from build123d import *

# Parameters (mm, degrees)
SKETCH1_W                  = 50.8
SKETCH1_H                  = 63.5
BOSS_EXTRUDE1_DEPTH        = 12.7
F_22_0_22_DIAMETER_HOLE1_D = 22
F_4_40_TAPPED_HOLE1_D      = 2.2606
CUT_EXTRUDE1_DEPTH         = 43.597094971
CUT_EXTRUDE2_DEPTH         = 6.35


with BuildPart() as part:
    # Sketch1 → Boss-Extrude1 (new body)
    with BuildSketch(Plane(origin=(0, 0, 0), x_dir=(0, 0, -1), z_dir=(1, 0, 0))):
        Rectangle(SKETCH1_W, SKETCH1_H)
    extrude(amount=BOSS_EXTRUDE1_DEPTH)

    # Ø22.0 (22) Diameter Hole1 (through all)
    with Locations(Plane(origin=(12.7, 0, 0), x_dir=(0, 0, -1), z_dir=(1, 0, 0))):
        with Locations((0, -12.7)):
            Hole(F_22_0_22_DIAMETER_HOLE1_D / 2)

    # Sketch4 → 1/16 NPT Tapped Hole1 (revolve, cut)
    with BuildSketch(Plane.ZX.offset(12.7)):
        Polygon((0, 0), (0, 13.530685027), (3.0734, 11.684), (3.0734, 6.858), (3.762574096, 6.858), (3.9679118, 0), align=None)
    revolve(axis=Axis((-6.35, 12.7, 0), (1, 0, 0)), mode=Mode.SUBTRACT)

    # #4-40 Tapped Hole1 (through all)
    with Locations(Plane(origin=(12.7, 0, 0), x_dir=(0, 0, -1), z_dir=(1, 0, 0))):
        with Locations((-12.5, 12.7), (12.5, 12.7)):
            Hole(F_4_40_TAPPED_HOLE1_D / 2)

    # Sketch9 → Cut-Extrude1 (cut, through all)
    with BuildSketch(Plane(origin=(12.7, 0, 0), x_dir=(0, 0, -1), z_dir=(1, 0, 0))):
        with BuildLine():
            Line((-3.65, 2.54), (3.65, 2.54))
            ThreePointArc((3.65, 2.54), (8.140128061, 4.399871939), (10, 8.89))
            Line((10, 8.89), (10, 16.51))
            ThreePointArc((10, 16.51), (8.140128061, 21.000128061), (3.65, 22.86))
            Line((3.65, 22.86), (-3.65, 22.86))
            ThreePointArc((-3.65, 22.86), (-8.140128061, 21.000128061), (-10, 16.51))
            Line((-10, 16.51), (-10, 8.89))
            ThreePointArc((-10, 8.89), (-8.140128061, 4.399871939), (-3.65, 2.54))
        make_face()
    extrude(amount=-CUT_EXTRUDE1_DEPTH, mode=Mode.SUBTRACT)

    # Sketch10 → Cut-Extrude2 (cut)
    with BuildSketch(Plane(origin=(0, 0, 0), x_dir=(0, 0, -1), z_dir=(1, 0, 0))):
        with BuildLine():
            Line((-12.5, 2.54), (12.5, 2.54))
            ThreePointArc((12.5, 2.54), (16.990128061, 4.399871939), (18.85, 8.89))
            Line((18.85, 8.89), (18.85, 16.51))
            ThreePointArc((18.85, 16.51), (16.990128061, 21.000128061), (12.5, 22.86))
            Line((12.5, 22.86), (-12.5, 22.86))
            ThreePointArc((-12.5, 22.86), (-16.990128061, 21.000128061), (-18.85, 16.51))
            Line((-18.85, 16.51), (-18.85, 8.89))
            ThreePointArc((-18.85, 8.89), (-16.990128061, 4.399871939), (-12.5, 2.54))
        make_face()
    extrude(amount=CUT_EXTRUDE2_DEPTH, mode=Mode.SUBTRACT)


solid = part.part
Part model, mm, in its own coordinate system. A direction names the side the tool comes from. Round coordinates to 2 decimals unless told otherwise and drop trailing zeros. Write each loop counter-clockwise with the first axis right and the second up, starting at its lowest first coordinate (ties: lowest second). Pieces come first, ordered by that corner, then holes. Notation, with made-up numbers: M -18.5,-26.75 L 24.5,-26.75 A30 ccw 24.5,3.25 Z; hole C 80.25,10.25 d11. An arc over 180 degrees is marked long. Return JSON: item names as keys, results as strings. Group by question number.
(1) Saw through at C-C on x = 11.75. Write the cut outline in (y, z).
(2) Saw through at B-B on y = -12.7. Write the cut outline in (x, z).
(3) Pin check, flat tips, straight feed: pin 1 Ø10 at (y, z) = (12, -3) entering from -X; pin 2 Ø12 at (y, z) = (12, 8) entering from -X. Stop position of each tip, or through.
(4) Saw through at D-D on y = 12.7. Write the cut outline in (x, z), then the cut area to 3 significant figures.
(5) Drill centre lines: probe 1 along Y at (x, z) = (4.5, 0); probe 2 along Y at (x, z) = (9.5, 12.5); probe 3 along Y at (x, z) = (7.5, -1.5). Where is each one in solid material? Low to high.
(6) Saw through at A-A on z = 0. Write the cut outline in (x, y).
(7) Which spindle directions (+Z, -Z, +X, -X, +Y, -Y) get a long thin tool onto all of the face, cutting with end or side? Do faces 5 (the face through (3.13, 4.35, -16.94)), 6 (the face through (9.57, 21.05, 8.09)), 7 (the face through (0, 0, 0)). Say none if no direction does.
(8) Two-plate mould, pull along Z, no slides. Class faces 1 (the face through (6.35, 13, 15)), 2 (the face through (6, 31.75, 0)), 3 (the face through (6, 0, -25.4)), 4 (the face through (10, 13, -10)): +Z half, -Z half, draft (parallel to the pull), parting line (faces both ways), or undercut.
Returned:
{
 "1": {"outline": "M -31.75,-25.4 L 31.75,-25.4 L 31.75,25.4 L -31.75,25.4 Z; hole C -12.7,0 d22; hole M 2.54,-3.65 A6.35 ccw 8.89,-10 L 16.51,-10 A6.35 ccw 22.86,-3.65 L 22.86,3.65 A6.35 ccw 16.51,10 L 8.89,10 A6.35 ccw 2.54,3.65 Z; hole C 12.7,-12.5 d2.26; hole C 12.7,12.5 d2.26"},
 "2": {"outline": "M 0,-25.4 L 12.7,-25.4 L 12.7,-11 L 0,-11 Z; M 0,11 L 12.7,11 L 12.7,25.4 L 0,25.4 Z"},
 "3": {"pin 1": "through", "pin 2": "x = 6.35"},
 "4": {"outline": "M 0,-25.4 L 12.7,-25.4 L 12.7,-13.63 L 6.35,-13.63 L 6.35,-18.85 L 0,-18.85 Z; M 0,18.85 L 6.35,18.85 L 6.35,13.63 L 12.7,13.63 L 12.7,25.4 L 0,25.4 Z; M 6.35,-11.37 L 12.7,-11.37 L 12.7,-10 L 6.35,-10 Z; M 6.35,10 L 12.7,10 L 12.7,11.37 L 6.35,11.37 Z", "area": "250 mm²"},
 "5": {"probe 1": "-31.75 to -23.7, -1.7 to 2.54, 22.86 to 31.75", "probe 2": "-31.75 to 11.57, 13.83 to 31.75", "probe 3": "-31.75 to -23.6, -1.8 to 2.54, 22.86 to 31.75"},
 "6": {"outline": "M 0,-31.75 L 12.7,-31.75 L 12.7,-23.7 L 0,-23.7 Z; M 0,-1.7 L 12.7,-1.7 L 12.7,2.54 L 0,2.54 Z; M 0,22.86 L 12.7,22.86 L 12.7,31.75 L 0,31.75 Z"},
 "7": {"face 5": "-X", "face 6": "+X, -X", "face 7": "+Z, -Z, -X, +Y, -Y"},
 "8": {"face 1": "undercut", "face 2": "draft", "face 3": "-Z half", "face 4": "undercut"}
}
